Autodesk Inventor part; units mm, degrees
ref_plane "Work Plane1" through (-7, 0, 0) normal (0, 1, 0) x (1, 0, 0)
ref_plane "YZ Plane" through (0, 0, 0) normal (1, 0, 0) x (0, 1, 0)
ref_plane "XZ Plane" through (0, 0, 0) normal (0, 1, 0) x (-1, 0, 0)
sketch "Sketch1" plane through (0, 0, 0) normal (0, 0, 1) x (1, 0, 0)
  circle A0 centre (0, 0) radius 2.25
  circle A1 centre (40, 0) radius 2.25
  line L0 (-7, 10) -> (47, 10)
  line L1 (-7, -10) -> (47, -10)
  line L2 (-7, -10) -> (-7, 10)
  line L3 (47, 10) -> (47, -10)
  dimension "d0" = 4.5
  dimension "d1" = 4.5
  dimension "d2" = 40
  dimension "d48" = 7
  dimension "d49" = 7
  dimension "d50" = 20
  dimension "d51" = 10
extrude "Extrusion1" add sketch "Sketch1" along normal blind 4
ref_plane "Work Plane1" through (-7, 0, 0) normal (0, 1, 0) x (1, 0, 0)
sketch "Sketch4" plane through (-7, 0, 0) normal (0, 1, 0) x (1, 0, 0)
  line L0 (0, 0) -> (54, 0)
  line L1 (0, 0) -> (0, -4)
  line L2 (54, -4) -> (0, -4)
  line L3 (54, 0) -> (54, -4)
  line L4 (0, 0) -> (0, 0)
  line L5 (0, 0) -> (0, -4)
  line L6 (0, -4) -> (0, -4)
  line L7 (0, 0) -> (0, -4)
  line L8 (40, 0) -> (40, 0)
  line L9 (40, 0) -> (40, -4)
  line L10 (40, -4) -> (40, -4)
  line L11 (40, 0) -> (40, -4)
  circle A0 centre (27, -10) radius 5.1
  line L12 (14, -4) -> (14, -10)
  line L13 (14, -10) -> (21.9, -10)
  line L14 (32.1, -10) -> (40, -10)
  line L15 (40, -10) -> (40, -4)
  line L16 (0, -4) -> (54, -4)
  line L17 (14, -4) -> (40, -4)
  point P0 (7, 0)
  dimension "d23" = 10.2
  dimension "d24" = 6
  dimension "d25" = 26
  dimension "d26" = 13
  dimension "d27" = 14
extrude "Extrusion4" add sketch "Sketch4" along normal mid plane 20 contours L15 L14 A0 L13 L12 L2
chamfer "Chamfer1" distance 4 angle 45 2 edges at (7, 0, 4) (33, 0, 4)
sketch "Sketch5" plane through (0, 0, 4) normal (0, 0, 1) x (1, 0, 0)
  circle A0 centre (40, 0) radius 2.25
  line L0 (3, 10) -> (-7, 10)
  line L1 (-7, -10) -> (3, -10)
  circle A1 centre (0, 0) radius 2.25
  circle A2 centre (0, 0) radius 5
  circle A3 centre (40, 0) radius 2.25
  circle A4 centre (40, 0) radius 5
  circle A5 centre (40, 0) radius 2.25
  line L2 (47, -10) -> (47, 10)
  line L3 (47, 10) -> (37, 10)
  line L4 (-7, 10) -> (-7, -10)
  line L5 (37, -10) -> (37, 10)
  line L6 (37, -10) -> (47, -10)
  line L7 (3, 10) -> (3, -10)
  point P0 (39.5, -2.4495)
  point P1 (39.5, 2.4495)
  dimension "d33" = 10
  dimension "d34" = 10
extrude "Extrusion5" cut sketch "Sketch5" along normal up to surface (6 mm away) contours L7 A2 | A2 L7 | A1 | A4 L5 | L5 A4
sketch "Sketch6" plane through (7, 10, 10) normal (0, 0, 1) x (1, 0, 0)
  line L0 (26, -20) -> (26, 0)
  line L1 (18.1, 0) -> (26, 0)
  line L2 (18.1, -20) -> (18.1, 0)
  line L3 (26, -20) -> (18.1, -20)
  circle A0 centre (4, -10) radius 2
  circle A1 centre (22, -10) radius 2
  point P0 (-7, -10)
  dimension "d37" = 4
  dimension "d38" = 4
  dimension "d39" = 10
  dimension "d40" = 18
  dimension "d41" = 3.9
extrude "Extrusion6" cut sketch "Sketch6" against normal up to surface (10 mm away) contours A0 | A1
sketch "Sketch7" plane through (0, 0, 0) normal (0, 0, -1) x (-1, 0, 0)
  circle A0 centre (-11, 0) radius 2
  circle A1 centre (-29, 0) radius 2
  line L0 (-29, 4.2724) -> (-25.3, 2.1362)
  line L1 (-25.3, 2.1362) -> (-25.3, -2.1362)
  line L2 (-25.3, -2.1362) -> (-29, -4.2724)
  line L3 (-29, -4.2724) -> (-32.7, -2.1362)
  line L4 (-32.7, -2.1362) -> (-32.7, 2.1362)
  line L5 (-32.7, 2.1362) -> (-29, 4.2724)
  line L6 (-11, 4.2724) -> (-7.3, 2.1362)
  line L7 (-7.3, 2.1362) -> (-7.3, -2.1362)
  line L8 (-7.3, -2.1362) -> (-11, -4.2724)
  line L9 (-11, -4.2724) -> (-14.7, -2.1362)
  line L10 (-14.7, -2.1362) -> (-14.7, 2.1362)
  line L11 (-14.7, 2.1362) -> (-11, 4.2724)
  dimension "d44" = 7.4
extrude "Extrusion7" cut sketch "Sketch7" against normal blind 3.5
chamfer "Chamfer2" distance 4 angle 45 4 edges at (-7, 10, 2) (-7, -10, 2) (47, 10, 2) (47, -10, 2)
properties part number "ZAxisRodClampBody" material "ABS Plastic"
Geometry check sheet. Reference: the model listing, model coordinates, mm. A direction names the side the tool comes from. Round coordinates to 2 decimals unless told otherwise and drop trailing zeros. Write each loop counter-clockwise with the first axis right and the second up, starting at its lowest first coordinate (ties: lowest second). Pieces come first, ordered by that corner, then holes. Notation, with made-up numbers: (-28, 46.5) -> (4, 46.5) arc R27 cw to (4, 68.5) -> close; hole circle Ø11 at (-7.75, -38). An arc over 180 degrees is marked (long way). Put each result on its own line as item: value.
1) Cross-section at B-B, the plane y = -6.5. Enter the section's corners in (x, z), plus the area to 3 significant figures.
Recorded:
outline: (-6.5, 0) -> (46.5, 0) -> (46.5, 4) -> (37, 4) -> (33, 8) -> (33, 10) -> (25.1, 10) arc R5.1 cw to (14.9, 10) -> (7, 10) -> (7, 8) -> (3, 4) -> (-6.5, 4) -> close
area: 343 mm2
2) Cross-section at A-A, the plane x = 36. Enter the section's corners in (y, z), plus the area to 3 significant figures.
Recorded:
outline: (-10, 0) -> (10, 0) -> (10, 5) -> (3, 5) -> (3, 4) -> (-3, 4) -> (-3, 5) -> (-10, 5) -> close
area: 94.0 mm2
3) Depth check by flat-ended pin: P1, Ø9.5, axis at x = 43.5, y = 3.5, coming from the +Z side; P2, Ø1, axis at y = -2, z = 9, coming from the +X side; P3, Ø0.6, axis at y = -2.5, z = 9.5, coming from the -X side. Enter the tip coordinate at first touch or a pass-through.
Recorded:
P1: stops at z = 4
P2: stops at x = 33
P3: stops at x = 7
4) Cross-section at C-C, the plane z = 2.25. Enter the section's corners in (x, y).
Recorded:
outline: (-7, -6) -> (-3, -10) -> (43, -10) -> (47, -6) -> (47, 6) -> (43, 10) -> (-3, 10) -> (-7, 6) -> close; hole circle Ø4.5 at (0, 0); hole (7.3, -2.14) -> (11, -4.27) -> (14.7, -2.14) -> (14.7, 2.14) -> (11, 4.27) -> (7.3, 2.14) -> close; hole (25.3, -2.14) -> (29, -4.27) -> (32.7, -2.14) -> (32.7, 2.14) -> (29, 4.27) -> (25.3, 2.14) -> close; hole circle Ø4.5 at (40, 0)
5) Release check for a two-part mould opening along X. For faces 5 (the face through (20, 0, 0)), 6 (the face through (30.908, 0.601, 6.796)), 7 (the face through (47, 0, 2)) record: pulls with the +X half, pulls with the -X half, needs draft (parallel to the pull), parting line crosses it, or undercut.
Recorded:
face 5: needs draft
face 6: undercut
face 7: pulls with the +X half
6) Thickness scan on probe 1 along X at (y, z) = (-0.25, 4.5); probe 2 along X at (y, z) = (0.25, 3); probe 3 along Y at (x, z) = (0, 1.5). Record the ranges inside material, lowest first. Write a range as from..to.
Recorded:
probe 1: x = 4.99..9.02, 12.98..27.02, 30.98..35.01
probe 2: x = -7..-2.24, 2.24..7.3, 14.7..25.3, 32.7..37.76, 42.24..47
probe 3: y = -10..-2.25, 2.25..10
7) Access from +Z, -Z, +X, -X, +Y, -Y to the whole of each face (thin tool, end or side, straight path). Record for faces 1 (the face through (33, 0, 9)), 2 (the face through (35, 0, 5)), 3 (the face through (27.18, 3.22, 1.73)), 4 (the face through (37.752, -0.099, 1.972)).
Recorded:
face 1: +Z, +X, +Y, -Y
face 2: +Z, +X
face 3: -Z
face 4: +Z, -Z
8) Cross-section at D-D, the plane y = 0. Give the number of separate pieces and of enclosed holes in the cut face, plus the area to 3 significant figures.
Recorded:
separate pieces: 5
enclosed holes: 0
area: 203 mm2
